Geometry: final body of the model. Coordinates: model frame, mm. Face numbers are marked on the shaded views. A direction names the side the tool comes from. Round coordinates to 2 decimals unless told otherwise and drop trailing zeros. Order: outer loops, then holes, each group sorted by start corner. A loop starts at its lowest first (then second) coordinate and runs counter-clockwise, first axis right, second up. Notation, with made-up numbers: (86.5, 82.25) - (145.5, 82.25) arc R27 cw to (145.5, 117.25) - close; hole circle Ø6 at (-13, 31). An arc over 180 degrees is marked (long way). Put each result on its own line as item: value. Start each with the question number.
(1) Material intervals for L1, parallel to Y at x = -12.25, z = -27.5; L2, parallel to Z at x = -5.5, y = 0; L3, parallel to Z at x = -12.5, y = 0, sorted ascending. Write a range as [from, to].
(2) Section B-B (z = 8). Output: boundary loops of the cut face in (x, y).
(3) Section D-D (x = -6.5). Output: boundary loops of the cut face in (y, z), and give its area (3 significant figures).
(4) Pin query (flat end, axial travel): P1, Ø2, axis at y = -1.5, z = -28, coming from the +X side; P2, Ø6, axis at y = 0, z = -27.5, coming from the -X side; P3, Ø2, axis at x = -9.5, y = -6, coming from the -Z side; P4, Ø3, axis at x = -6.5, y = 2.5, coming from the +Z side. Return the tip coordinate at first contact, or that it passes through.
(5) Section C-C (x = -1.5). Output: boundary loops of the cut face in (y, z) (1 decimal).
(6) Pull-direction query (Z, two-part tool) for the marked faces 3, 4 and 5; classes: released by +Z, released by -Z, zero draft, split by the parting line, or undercut.
(7) Access query for the marked faces 1 and 2. Directions: +Z, -Z, +X, -X, +Y, -Y. A direction counts if a zero-diameter tool reaches every point of the face in a straight line with its end or side. Return the directions, or none.
(8) Section A-A (x = -13). Output: boundary loops of the cut face in (y, z).
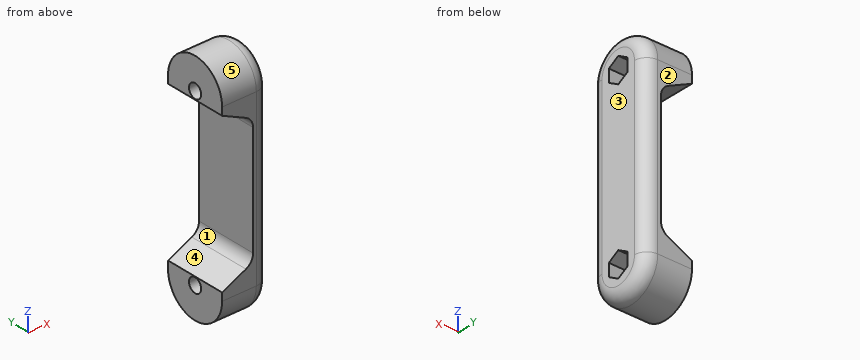
Autodesk Inventor part; units mm, degrees
ref_plane "YZ Plane" through (0, 0, 0) normal (1, 0, 0) x (0, 1, 0)
ref_plane "XZ Plane" through (0, 0, 0) normal (0, 1, 0) x (-1, 0, 0)
ref_plane "XY Plane" through (0, 0, 0) normal (0, 0, 1) x (1, 0, 0)
sketch "Sketch1" plane through (0, 0, 0) normal (1, 0, 0) x (0, 1, 0)
  line L0 (10, 37.5) -> (-10, 37.5)
  line L1 (-10, 37.5) -> (-10, -37.5)
  line L2 (-10, -37.5) -> (10, -37.5)
  line L3 (10, -37.5) -> (10, 37.5)
  line L4 (10, 37.5) -> (-10, -37.5) construction
  line L5 (-10, 37.5) -> (10, -37.5) construction
  circle A0 centre (0, 27.5) radius 10
  circle A1 centre (0, -27.5) radius 10
  point P0 (0, 0)
  point P1 (10, -27.5)
  point P2 (10, 27.5)
  point P3 (-10, 27.5)
  point P4 (-10, -27.5)
  dimension "d0" = 20
  dimension "d1" = 75
  dimension "d2" = 20
  dimension "d3" = 20
  dimension "d4" = 55
extrude "Extrusion1" add sketch "Sketch1" against normal blind 15 contours A0 | L3 A1 L1 A0 | A1
sketch "Sketch2" plane through (0, -10, -27.5) normal (0, -1, 0) x (1, 0, 0)
  line L0 (-15, 55) -> (-15, 0)
  line L1 (-15, 52.5125) -> (-5.0401, 47.8284)
  line L2 (-5.0401, 47.8284) -> (-5.0401, 7.1716)
  line L3 (-5.0401, 7.1716) -> (-15, 2.4875)
  line L4 (-15, 0) -> (-15, -10)
  line L5 (0, 55) -> (0, 65) construction
  line L6 (0, 65) -> (-5.0401, 47.8284) construction
  line L7 (0, -10) -> (0, 0) construction
  line L8 (-5.0401, 7.1716) -> (0, -10) construction
  point P0 (0, 27.5)
  point P1 (-15, 2.4875)
extrude "Extrusion2" cut sketch "Sketch2" against normal blind 20
fillet "Fillet1" radius 4 6 edges at (0, -10, 0) (0, 0, -37.5) (0, 10, 0) (0, 0, 37.5) (-5.0401, 0, -20.3284) (-5.0401, 0, 20.3284)
sketch "Sketch3" plane through (0, 0, 0) normal (1, 0, 0) x (0, 0, -1)
  line L0 (25.0125, -10) -> (25.0125, 10)
  line L1 (25.0125, 10) -> (27.5, 10)
  arc A0 (27.5, -10) -> (27.5, 10) centre (27.5, 0) ccw
  line L2 (27.5, -10) -> (25.0125, -10)
  arc A1 (-27.5, 6) -> (-27.5, -6) centre (-27.5, 0) ccw
  line L3 (-23.4585, 0) -> (-25.4793, -3.5)
  line L4 (-25.4793, -3.5) -> (-29.5207, -3.5)
  line L5 (-29.5207, -3.5) -> (-31.5415, 0)
  line L6 (-31.5415, 0) -> (-29.5207, 3.5)
  line L7 (-29.5207, 3.5) -> (-25.4793, 3.5)
  line L8 (-25.4793, 3.5) -> (-23.4585, 0)
  line L9 (23.4585, 0) -> (25.4793, 3.5)
  line L10 (25.4793, 3.5) -> (29.5207, 3.5)
  line L11 (29.5207, 3.5) -> (31.5415, 0)
  line L12 (31.5415, 0) -> (29.5207, -3.5)
  line L13 (29.5207, -3.5) -> (25.4793, -3.5)
  line L14 (25.4793, -3.5) -> (23.4585, 0)
  point P0 (0, 0)
  dimension "d10" = 7
  dimension "d11" = 7
extrude "Extrusion3" cut sketch "Sketch3" against normal blind 10 contours L14 L9 L0 | L0 L9 L10 L11 L12 L13 L14 | L3 L4 L5 L6 L7 L8
sketch "Sketch4" plane through (-15, 0, 0) normal (-1, 0, 0) x (0, 0, 1)
  line L0 (-21.409, 10) -> (-21.409, -10)
  line L1 (-29.5207, 3.5) -> (-31.5415, 0)
  line L2 (-31.5415, 0) -> (-29.5207, -3.5)
  line L3 (-29.5207, -3.5) -> (-25.4793, -3.5)
  line L4 (-25.4793, -3.5) -> (-23.4585, 0)
  line L5 (-23.4585, 0) -> (-25.4793, 3.5)
  line L6 (-25.4793, 3.5) -> (-29.5207, 3.5)
  line L7 (29.5207, 3.5) -> (25.4793, 3.5)
  line L8 (25.4793, 3.5) -> (23.4585, 0)
  line L9 (23.4585, 0) -> (25.4793, -3.5)
  line L10 (25.4793, -3.5) -> (29.5207, -3.5)
  line L11 (29.5207, -3.5) -> (31.5415, 0)
  line L12 (31.5415, 0) -> (29.5207, 3.5)
  line L13 (-27.5, -6) -> (27.5, -6)
  arc A0 (-27.5, 6) -> (-27.5, -6) centre (-27.5, 0) ccw
  line L14 (27.5, 6) -> (-27.5, 6)
  arc A1 (27.5, -6) -> (27.5, 6) centre (27.5, 0) ccw
  point P0 (0, 0)
hole "Hole1" at (-15, 0, -27.5) at (-15, 0, 27.5) direction (1, 0, 0) diameter 4.5 end through all
equation "\"d11\" = d10"
properties part number "controlbox_handvat"
Checks:
1. L1: y = [-10, -2.25], [2.25, 10]
1. L2: z = [-37.5, -31.54], [-23.46, -19.65], [19.65, 23.46], [31.54, 37.5]
1. L3: z = [-37.5, -29.75], [-25.25, -23.84], [23.84, 25.25], [29.75, 37.5]
2. outline: (-5.04, -10) - (-4, -10) arc R4 ccw to (0, -6) - (0, 6) arc R4 ccw to (-4, 10) - (-5.04, 10) - close
3. outline: (-10, -27.5) arc R10 ccw to (10, -27.5) - (10, -20.88) - (-10, -20.88) - close; (-10, 20.88) - (10, 20.88) - (10, 27.5) arc R10 ccw to (-10, 27.5) - close; hole (-3.5, -29.52) - (0, -31.54) - (3.5, -29.52) - (3.5, -25.48) - (0, -23.46) - (-3.5, -25.48) - close; hole (-3.5, 25.48) - (0, 23.46) - (3.5, 25.48) - (3.5, 29.52) - (0, 31.54) - (-3.5, 29.52) - close
3. area: 494 mm²
4. P1: stops at x = -10
4. P2: stops at x = -15
4. P3: stops at z = -36.16
4. P4: stops at z = 37.45
5. outline: (-9.1, -27.5) arc R9.1 ccw to (9.1, -27.5) - (9.1, 27.5) arc R9.1 ccw to (-9.1, 27.5) - close; hole (-3.5, -29.5) - (0, -31.5) - (3.5, -29.5) - (3.5, -25.5) - (0, -23.5) - (-3.5, -25.5) - close; hole (-3.5, 25.5) - (0, 23.5) - (3.5, 25.5) - (3.5, 29.5) - (0, 31.5) - (-3.5, 29.5) - close
6. face 3: zero draft
6. face 4: undercut
6. face 5: released by +Z
7. face 1: -X, +Y, -Y
7. face 2: +Z, -Z, +X, -X, +Y
8. outline: (-10, -27.5) arc R10 ccw to (10, -27.5) - (10, -24.07) - (-10, -24.07) - close; (-10, 24.07) - (10, 24.07) - (10, 27.5) arc R10 ccw to (-10, 27.5) - close; hole circle Ø4.5 at (0, -27.5); hole circle Ø4.5 at (0, 27.5)
